```python
from build123d import *

# Parameters (mm, degrees)
BOX021_W            = 10
BOX021_H            = 20
BOX021_DEPTH        = 10
BOX022_W            = 10
BOX022_H            = 20
BOX022_DEPTH        = 10
PAD007_DEPTH        = 1
BOX023_W            = 14
BOX023_H            = 20
BOX023_DEPTH        = 10
SKETCH007_W         = 4
SKETCH007_H         = 6
PAD006_DEPTH        = 1
CLONE008_ROLL_ANGLE = 90
CLONE009_ROLL_ANGLE = 90
PAD005_DEPTH        = 8
CLONE007_ROLL_ANGLE = 90


with BuildPart() as cubo021:
    # Box021 → Box021 (new body)
    with BuildSketch(Plane(origin=(7.4, -10, -16), x_dir=(1, 0, 0), z_dir=(0, 0, 1))):
        with Locations((5, 10)):
            Rectangle(BOX021_W, BOX021_H)
    extrude(amount=BOX021_DEPTH)


with BuildPart() as cubo022:
    # Box022 → Box022 (new body)
    with BuildSketch(Plane(origin=(-17.4, -10, -16), x_dir=(1, 0, 0), z_dir=(0, 0, 1))):
        with Locations((5, 10)):
            Rectangle(BOX022_W, BOX022_H)
    extrude(amount=BOX022_DEPTH)


with BuildPart() as cut034:
    # Sketch008 → Pad007 (new body)
    with BuildSketch(Plane(origin=(0, 0, -12.6), x_dir=(-1, 0, 0), z_dir=(0, 0, 1))):
        with BuildLine():
            add(Edge.make_bspline(
                [(8.550522, 0), (8.550522, 13.423394), (-4.275261, 6.711697), (-17.101044, 0), (-4.275261, -6.711697), (8.550522, -13.423394), (8.550522, 0)],
                knots=[0, 0, 0, 2.094395, 2.094395, 4.18879, 4.18879, 6.283185, 6.283185, 6.283185], degree=2, weights=[1, 0.5, 1, 0.5, 1, 0.5, 1]))
        make_face()
        with BuildLine():
            ThreePointArc((4.444579, 3.239709), (-5.5, 0), (4.444579, -3.239709))
            Line((4.444579, -3.239709), (4.444579, 3.239709))
        make_face(mode=Mode.SUBTRACT)
    extrude(amount=PAD007_DEPTH)

    # Cut033: cut Cubo022
    add(cubo022.part, mode=Mode.SUBTRACT)

    # Cut034: cut Cubo021
    add(cubo021.part, mode=Mode.SUBTRACT)


with BuildPart() as cubo023:
    # Box023 → Box023 (new body)
    with BuildSketch(Plane(origin=(-7, -10, -16), x_dir=(1, 0, 0), z_dir=(0, 0, 1))):
        with Locations((7, 10)):
            Rectangle(BOX023_W, BOX023_H)
    extrude(amount=BOX023_DEPTH)


with BuildPart() as obj1:
    # Sketch007 → Pad006 (new body)
    with BuildSketch(Plane.YZ):
        with BuildLine():
            Line((-3.5, 6), (3.5, 6))
            ThreePointArc((4.5, 5), (4.207107, 5.707107), (3.5, 6))
            ThreePointArc((4.488917, -5.148471), (5.130693, -0.074931), (4.5, 5))
            ThreePointArc((3.5, -6), (4.152506, -5.757783), (4.488917, -5.148471))
            Line((3.5, -6), (-3.5, -6))
            ThreePointArc((-4.5, -5), (-4.207107, -5.707107), (-3.5, -6))
            Line((-4.5, -5), (-4.5, 5))
            ThreePointArc((-3.5, 6), (-4.207107, 5.707107), (-4.5, 5))
        make_face()
        with Locations((0.5, 0)):
            Rectangle(SKETCH007_W, SKETCH007_H, mode=Mode.SUBTRACT)
    extrude(amount=PAD006_DEPTH)


with BuildPart() as obj2:
    # Clone008 base: copy of obj1
    add(obj1.part)


with BuildPart() as obj2_1:
    # Clone008 roll: moved
    add(obj2.part.rotate(Axis((0, 0, 0), (1, 0, 0)), CLONE008_ROLL_ANGLE))


with BuildPart() as obj2_2:
    # Clone008 placement: moved
    add(obj2_1.part.moved(Location((-10.1, 0, 4.29))))


with BuildPart() as obj3:
    # Clone009 base: copy of obj1
    add(obj1.part)


with BuildPart() as obj3_1:
    # Clone009 roll: moved
    add(obj3.part.rotate(Axis((0, 0, 0), (1, 0, 0)), CLONE009_ROLL_ANGLE))


with BuildPart() as obj3_2:
    # Clone009 placement: moved
    add(obj3_1.part.moved(Location((9.1, 0, 4.29))))


with BuildPart() as brida:
    # Sketch006 → Pad005 (new body)
    with BuildSketch(Plane.XY):
        with BuildLine():
            Line((-10.1, 0.787419), (-9.1, 0.787419))
            Line((-9.1, 0.787419), (-9.1, -9.212581))
            ThreePointArc((-9.1, -9.212581), (-8.367767, -10.980348), (-6.6, -11.712581))
            Line((-6.6, -11.712581), (6.6, -11.712581))
            ThreePointArc((6.6, -11.712581), (8.367767, -10.980348), (9.1, -9.212581))
            Line((9.1, -9.212581), (9.1, 0.787419))
            Line((9.1, 0.787419), (10.1, 0.787419))
            Line((10.1, 0.787419), (10.1, -9.212581))
            ThreePointArc((6.6, -12.712581), (9.074874, -11.687455), (10.1, -9.212581))
            Line((6.6, -12.712581), (-6.6, -12.712581))
            ThreePointArc((-10.1, -9.212581), (-9.074874, -11.687455), (-6.6, -12.712581))
            Line((-10.1, -9.212581), (-10.1, 0.787419))
        make_face()
    extrude(amount=PAD005_DEPTH)


with BuildPart() as brida_1:
    # Clone007 roll: moved
    add(brida.part.rotate(Axis((0, 0, 0), (1, 0, 0)), CLONE007_ROLL_ANGLE))


with BuildPart() as brida_2:
    # Clone007 placement: moved
    add(brida_1.part.moved(Location((0, 4, 0))))

    # Fusion014: union obj2, obj3
    add(obj2_2.part)
    add(obj3_2.part)

    # Cut032: cut Cubo023
    add(cubo023.part, mode=Mode.SUBTRACT)

    # Fusion015: union Cut034
    add(cut034.part)


with BuildPart() as brida_3:
    # Fusion015 placement: moved
    add(brida_2.part.moved(Location((8.6, 11.25, -13.6))))


solid = brida_3.part
```
Could you check a few things on this model? Use its own coordinates, in mm. A direction names the side the tool comes from. Round coordinates to 2 decimals unless told otherwise and drop trailing zeros. Loops run counter-clockwise (first coordinate to the right, second up) from the corner with the lowest first, then second, coordinate; pieces in that order, holes last. Notation, with made-up numbers: (18.25, 49) - (36.25, 49) arc R15 cw to (36.25, 76) - close; hole circle Ø6 at (89, 53.25). An arc over 180 degrees is marked (long way). Answer in a Markdown table with one row per item. Add a question column.
(1) If we section it at C-C (x = 16.75): Please give me the cut outline in (y, z).
(2) I need wall thicknesses on line 1 along Y through (x, z) = (8.6, -25.9); line 2 along X through (y, z) = (8.75, -18.5); line 3 along Z through (x, y) = (12, 17). Which ranges of each line are inside material? Lowest first, please.
(3) If we section it at B-B (y = 9.5): Please give me the cut outline in (x, z).
(4) If we section it at A-A (y = 11.5): Please give me the cut outline in (x, z).
(5) I'm going to push flat-ended pins straight in: pin 1 (4 mm diameter, centred on x = 15.5, y = 17, fed in from -Z); pin 2 (0.5 mm diameter, centred on x = -1, z = -9, fed in from -Y); pin 3 (10 mm diameter, centred on x = 10, z = -11.5, fed in from -Y); pin 4 (1.5 mm diameter, centred on x = 2, y = 16, fed in from -Z). Where does each tip first touch, or does it pass through?
(6) For faces 1 (the face through (4, 11, -25.2)), 2 (the face through (18, 8.25, -9)), 3 (the face through (18.193, 17.014, -5.165)), which set-ups out of +Z, -Z, +X, -X, +Y, -Y let a thin tool reach every point of the face, with its end or its side?
(7) If we mould it in two halves opening along Z, with no side actions, what happens to faces 4 (the face through (-1.01, 11.4, -4.18)), 5 (the face through (-1, 7.25, -20)), 6 (the face through (18, 11, -6.81))? For each: pulls with the +Z half, pulls with the -Z half, needs draft (parallel to the pull), parting line crosses it, or undercut.
(8) If we section it at D-D (y = 6.75): State how many separate pieces and enclosed holes the cut face has, plus the area to 3 significant figures.
Model answer:
| question | item | result |
|---|---|---|
| 1 | outline | (7.25, -25.95) - (15.25, -25.95) - (15.25, -24.77) - (7.25, -24.77) - close |
| 2 | line 1 | y = 3.5 to 5.75, 16.75 to 19 |
| 2 | line 2 | x = -1.5 to -0.5, 17.7 to 18.7 |
| 2 | line 3 | z = -26.2 to -25.2 |
| 3 | outline | (-1.5, -22.81) arc R3.5 ccw to (1.6, -26.29) - (1.6, -26.2) - (4.16, -26.2) - (4.16, -25.2) - (1.26, -25.2) arc R2.5 cw to (-0.5, -22.81) - (-0.5, -10.81) - (-1.5, -10.81) - close; (-1.5, -6.81) - (-0.5, -6.81) - (-0.5, -4.26) - (-1.5, -4.26) - close; (13.81, -26.2) - (15.6, -26.2) - (15.6, -26.29) arc R3.5 ccw to (18.7, -22.81) - (18.7, -10.81) - (17.7, -10.81) - (17.7, -22.81) arc R2.5 cw to (15.94, -25.2) - (13.81, -25.2) - close; (17.7, -6.81) - (18.7, -6.81) - (18.7, -4.26) - (17.7, -4.26) - close |
| 4 | outline | (-1.5, -22.81) arc R3.5 ccw to (1.6, -26.29) - (1.6, -26.2) - (4.16, -26.2) - (4.16, -25.2) - (1.26, -25.2) arc R2.5 cw to (-0.5, -22.81) - (-0.5, -10.81) - (-1.5, -10.81) - close; (-1.5, -6.81) - (-0.5, -6.81) - (-0.5, -4.18) - (-1.5, -4.18) - close; (14.09, -26.2) - (15.6, -26.2) - (15.6, -26.29) arc R3.5 ccw to (18.7, -22.81) - (18.7, -10.81) - (17.7, -10.81) - (17.7, -22.81) arc R2.5 cw to (15.94, -25.2) - (14.09, -25.2) - close; (17.7, -6.81) - (18.7, -6.81) - (18.7, -4.18) - (17.7, -4.18) - close |
| 5 | pin 1 | stops at z = -26.29 |
| 5 | pin 2 | stops at y = 5.25 |
| 5 | pin 3 | passes through |
| 5 | pin 4 | stops at z = -26.2 |
| 6 | face 1 | +Z, +Y, -Y |
| 6 | face 2 | +X, -X |
| 6 | face 3 | +Z, +X, -X, +Y |
| 7 | face 4 | pulls with the +Z half |
| 7 | face 5 | needs draft |
| 7 | face 6 | undercut |
| 8 | separate pieces | 4 |
| 8 | enclosed holes | 0 |
| 8 | area | 25.8 mm² |
